The model under review builds one solid part; all positions refer to its coordinate system, in mm. A direction names the side the tool comes from. Round coordinates to 2 decimals unless told otherwise and drop trailing zeros. Write each loop counter-clockwise with the first axis right and the second up, starting at its lowest first coordinate (ties: lowest second). Pieces come first, ordered by that corner, then holes. Notation, with made-up numbers: (66.5, -22) -> (107.5, -22) arc R22 ccw to (107.5, -3) -> close; hole circle Ø9 at (64.25, 35). An arc over 180 degrees is marked (long way). Answer in a Markdown table with one row per item. Add a question column.
```python
from build123d import *

# Parameters (mm, degrees)
SKETCH1_W                = 48.1838
SKETCH1_H                = 43.0276
BOSS_EXTRUDE1_DEPTH      = 9.8806
SKETCH2_W                = 1.9685
SKETCH2_H                = 8.2296
CUT_EXTRUDE1_DEPTH       = 66.350433821
SKETCH4_W                = 1.9685
SKETCH4_H                = 8.2296
CUT_EXTRUDE2_DEPTH       = 65.071479861
SKETCH7_W                = 2.93146275
SKETCH7_H                = 2.802785647
BOSS_EXTRUDE2_DEPTH      = 8.89
BOSS_EXTRUDE3_DEPTH      = 24.13
BOSS_EXTRUDE3_DEPTH_BACK = 24.13
SKETCH8_R                = 7.1247
SKETCH9_W                = 48.1838
SKETCH9_H                = 18.415
BOSS_EXTRUDE4_DEPTH      = 6.35
SKETCH10_R               = 10.536568217
BOSS_EXTRUDE5_DEPTH      = 18.0848
SKETCH11_R               = 10.588095361
BOSS_EXTRUDE6_DEPTH      = 18.0848
SKETCH12_W               = 3.635847489
SKETCH12_H               = 2.34172836
CUT_EXTRUDE3_DEPTH       = 79.754744187
SKETCH14_W               = 3.684147677
SKETCH14_H               = 13.068356619
CUT_EXTRUDE4_DEPTH       = 79.754744187
SKETCH15_R               = 14.605
BOSS_EXTRUDE7_DEPTH      = 4.6228
SKETCH16_R               = 11.8745
BOSS_EXTRUDE8_DEPTH      = 11.4808
SKETCH18_R               = 2.159
CUT_EXTRUDE5_DEPTH       = 11.4808
SKETCH19_W               = 29.0322
SKETCH19_H               = 23.8252
BOSS_EXTRUDE9_DEPTH      = 29.972
SKETCH20_W               = 5.701054359
SKETCH20_H               = 24.361747341
CUT_EXTRUDE6_DEPTH       = 29.972
SKETCH21_W               = 19.733319163
SKETCH21_H               = 0.544777799
BOSS_EXTRUDE10_DEPTH     = 7.62


with BuildPart() as part:
    # Sketch1 → Boss-Extrude1 (new body)
    with BuildSketch(Plane(origin=(0, 0, 0), x_dir=(1, 0, 0), z_dir=(0, 1, 0))):
        with Locations((24.0919, 21.5138)):
            Rectangle(SKETCH1_W, SKETCH1_H)
    extrude(amount=BOSS_EXTRUDE1_DEPTH)

    # Sketch2 → Cut-Extrude1 (cut, through all)
    with BuildSketch(Plane(origin=(48.1838, 0, 0), x_dir=(0, 0, -1), z_dir=(1, 0, 0))):
        with Locations((42.04335, 4.1148)):
            Rectangle(SKETCH2_W, SKETCH2_H)
        with Locations((0.98425, 4.1148)):
            Rectangle(SKETCH2_W, SKETCH2_H)
    extrude(amount=-CUT_EXTRUDE1_DEPTH, mode=Mode.SUBTRACT)

    # Sketch4 → Cut-Extrude2 (cut, through all)
    with BuildSketch(Plane.XY.offset(-1.9685)):
        with Locations((0.98425, 4.1148)):
            Rectangle(SKETCH4_W, SKETCH4_H)
        with Locations((47.19955, 4.1148)):
            Rectangle(SKETCH4_W, SKETCH4_H)
    extrude(amount=-CUT_EXTRUDE2_DEPTH, mode=Mode.SUBTRACT)

    # Sketch7 → Boss-Extrude2 (add)
    with BuildSketch(Plane(origin=(0, 9.8806, 0), x_dir=(1, 0, 0), z_dir=(0, 1, 0))):
        with Locations((25.557631375, 20.112407176)):
            Rectangle(SKETCH7_W, SKETCH7_H)
    extrude(amount=BOSS_EXTRUDE2_DEPTH)

    # Sketch8 → Boss-Extrude3 (add, two sides: drawn at the far end of the back side and taken through both)
    with BuildSketch(Plane.ZY.offset(-24.0919).offset(-BOSS_EXTRUDE3_DEPTH_BACK)):
        with Locations((-21.5138, 18.7706)):
            Circle(SKETCH8_R)
    extrude(amount=BOSS_EXTRUDE3_DEPTH + BOSS_EXTRUDE3_DEPTH_BACK)

    # Sketch9 → Boss-Extrude4 (add)
    with BuildSketch(Plane(origin=(0, 9.8806, 0), x_dir=(1, 0, 0), z_dir=(0, 1, 0))):
        with Locations((24.0919, 21.5138)):
            Rectangle(SKETCH9_W, SKETCH9_H)
    extrude(amount=BOSS_EXTRUDE4_DEPTH)

    # Sketch10 → Boss-Extrude5 (add)
    with BuildSketch(Plane(origin=(48.2219, 0, 0), x_dir=(0, 0, -1), z_dir=(1, 0, 0))):
        with Locations((21.5138, 18.7706)):
            Circle(SKETCH10_R)
    extrude(amount=BOSS_EXTRUDE5_DEPTH)

    # Sketch11 → Boss-Extrude6 (add)
    with BuildSketch(Plane.ZY.offset(0.0381)):
        with Locations((-21.5138, 18.7706)):
            Circle(SKETCH11_R)
    extrude(amount=BOSS_EXTRUDE6_DEPTH)

    # Sketch12 → Cut-Extrude3 (cut, through all)
    with BuildSketch(Plane.XY.offset(-12.3063)):
        with Locations((25.909823745, 11.05146418)):
            Rectangle(SKETCH12_W, SKETCH12_H)
    extrude(amount=-CUT_EXTRUDE3_DEPTH, mode=Mode.SUBTRACT)

    # Sketch14 → Cut-Extrude4 (cut, through all)
    with BuildSketch(Plane.XY.offset(-12.3063)):
        with Locations((25.933973839, 18.75650667)):
            Rectangle(SKETCH14_W, SKETCH14_H)
    extrude(amount=-CUT_EXTRUDE4_DEPTH, mode=Mode.SUBTRACT)

    # Sketch15 → Boss-Extrude7 (add)
    with BuildSketch(Plane(origin=(0, 9.8806, 0), x_dir=(1, 0, 0), z_dir=(0, 1, 0))):
        with Locations((24.0919, 21.5138)):
            Circle(SKETCH15_R)
    extrude(amount=BOSS_EXTRUDE7_DEPTH)

    # Sketch16 → Boss-Extrude8 (add)
    with BuildSketch(Plane(origin=(0, 14.5034, 0), x_dir=(1, 0, 0), z_dir=(0, 1, 0))):
        with Locations(Location((24.0919, 21.5138, 0), (0, 0, 50.84140908))):
            Circle(SKETCH16_R)
    extrude(amount=BOSS_EXTRUDE8_DEPTH)

    # Sketch18 → Cut-Extrude5 (cut)
    with BuildSketch(Plane(origin=(0, 9.8806, 0), x_dir=(1, 0, 0), z_dir=(0, 1, 0))):
        with Locations(Location((42.7228, 37.5666, 0), (0, 0, 270))):
            Circle(SKETCH18_R)
    extrude(amount=-CUT_EXTRUDE5_DEPTH, mode=Mode.SUBTRACT)

    # Sketch19 → Boss-Extrude9 (add)
    with BuildSketch(Plane.XZ):
        with Locations((25.0444, -21.5519)):
            Rectangle(SKETCH19_W, SKETCH19_H)
    extrude(amount=BOSS_EXTRUDE9_DEPTH)

    # Sketch20 → Cut-Extrude6 (cut)
    with BuildSketch(Plane.XY.offset(-9.6393)):
        with Locations((13.378827179, -13.505025304)):
            Rectangle(SKETCH20_W, SKETCH20_H)
    extrude(amount=-CUT_EXTRUDE6_DEPTH, mode=Mode.SUBTRACT)

    # Sketch21 → Boss-Extrude10 (add)
    with BuildSketch(Plane.ZY.offset(-10.5283)):
        with Locations((-21.607385296, -27.502260314)):
            Rectangle(SKETCH21_W, SKETCH21_H)
    extrude(amount=BOSS_EXTRUDE10_DEPTH)


solid = part.part
```
1. For L1, parallel to Y at x = 20.5, z = -33; L2, parallel to Y at x = 20.5, z = -32; L3, parallel to X at y = 6, z = -18.5, list the stretches that pass through material, from the lowest coordinate up.
2. Add section C-C on x = 27. Write out the cut boundary in (y, z), plus the area to 3 significant figures.
3. Insertion check: pin 1 Ø3 at (x, z) = (-9, -13) entering from -Y; pin 2 Ø8 at (y, z) = (-12, -38) entering from -X; pin 3 Ø1.3 at (x, z) = (12, -13.5) entering from +Y; pin 4 Ø12 at (x, z) = (46, -6.5) entering from +Y. Each pin has a flat end and moves straight along its axis. Give the tip position at first contact, or say it passes through.
4. Add section B-B on y = -18. Write out the cut boundary in (x, z), plus the area to 3 significant figures.
5. Tool access review of faces 4 (the flat face through (16.229, -14, -21)), 5 (the cylindrical face through (-8.954, 8.434, -23.809)), 6 (the flat face through (-0.038, 21.3, -14.6)), 7 (the flat face through (6, 13, -30.721)), 8 (the flat face through (6, 13, -12.306)): name each direction out of +Z, -Z, +X, -X, +Y, -Y from which nothing blocks a thin tool from reaching the whole face with its end or side.
6. Add section D-D on y = 4.5. Write out the cut boundary in (x, z).
7. Add section A-A on z = -3.5. Write out the cut boundary in (x, y), plus the area to 3 significant figures.
8. Mouldability with a two-part tool opening along Y and no side actions: class faces 1 (the flat face through (25, -29.972, -21)), 2 (the flat face through (10.528, -28, -22)), 3 (the flat face through (24, 4, -1.968)) as pulls with the +Y half, pulls with the -Y half, needs draft (parallel to the pull), parting line crosses it, or undercut.
Filled in:
| question | item | result |
|---|---|---|
| 1 | L1 | -29.97 to 14.5 |
| 1 | L2 | -29.97 to 25.98 |
| 1 | L3 | 1.97 to 46.22 |
| 2 | outline | (-29.97, -33.46) -> (0, -33.46) -> (0, -41.06) -> (8.23, -41.06) -> (8.23, -43.03) -> (9.88, -43.03) -> (9.88, -35.83) -> (14.5, -35.83) -> (14.5, -33.03) -> (25.98, -33.03) -> (25.98, -10) -> (14.5, -10) -> (14.5, -7.2) -> (9.88, -7.2) -> (9.88, 0) -> (8.23, 0) -> (8.23, -1.97) -> (0, -1.97) -> (0, -9.64) -> (-29.97, -9.64) -> close |
| 2 | area | 1,500 mm² |
| 3 | pin 1 | y = 10.84 |
| 3 | pin 2 | through |
| 3 | pin 3 | y = 16.23 |
| 3 | pin 4 | y = 23.45 |
| 4 | outline | (16.23, -33.46) -> (39.56, -33.46) -> (39.56, -9.64) -> (16.23, -9.64) -> close |
| 4 | area | 556 mm² |
| 5 | face 4 | +Z, -Z, -X |
| 5 | face 5 | -X |
| 5 | face 6 | none |
| 5 | face 7 | -Z, +Y |
| 5 | face 8 | +Z, +Y |
| 6 | outline | (1.97, -41.06) -> (46.22, -41.06) -> (46.22, -1.97) -> (1.97, -1.97) -> close; hole circle Ø4.32 at (42.72, -37.57) |
| 7 | outline | (0, 8.23) -> (1.97, 8.23) -> (1.97, 0) -> (46.22, 0) -> (46.22, 8.23) -> (48.18, 8.23) -> (48.18, 9.88) -> (0, 9.88) -> close |
| 7 | area | 444 mm² |
| 8 | face 1 | pulls with the -Y half |
| 8 | face 2 | undercut |
| 8 | face 3 | needs draft |
